Print and shaded views of the part. All mm, measured from the part's lowest x, y and z. Round coordinates to 2 decimals unless told otherwise and drop trailing zeros. Order: outer loops, then holes, each group sorted by start corner. A loop starts at its lowest first (then second) coordinate and runs counter-clockwise, first axis right, second up. Notation, with made-up numbers: (-34, -15) - (-2, -15) arc R27 cw to (-2, 4) - close; hole circle Ø7 at (-0.5, -18). An arc over 180 degrees is marked (long way). Write item = value, one per line. Start each with the question number.
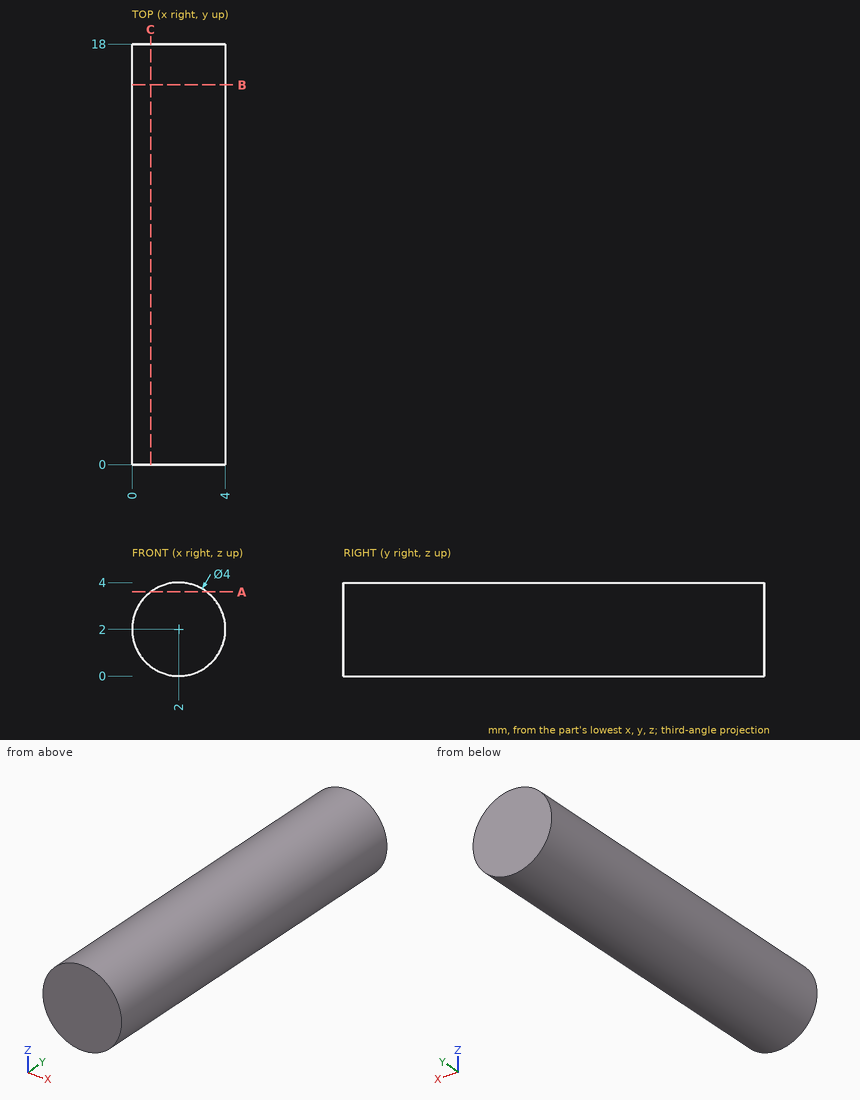
Item 1: Drop a flat-ended pin along its axis: pin 1 (2 mm diameter, centred on x = 0.5, y = 2, fed in from -Z). Give the stop position or say it passes through.
Item 2: Saw through at C-C, the plane x = 0.8. Give the cut face in (y, z), then the cut area to 3 significant figures.
Item 3: Saw through at B-B, the plane y = 16.25. Give the cut face in (x, z).
Item 4: Saw through at A-A, the plane z = 3.6. Give the cut face in (x, y).
Item 5: Probe L1, parallel to X at y = 16.25, z = 2.1; L2, parallel to Z at x = 0.65, y = 7.25; L3, parallel to Z at x = 2.5, y = 16. List the from-to ranges inside material, lowest first.
Check sheet entries:
q1.pin_1 = 0.06
q2.outline = (0, 0.4) - (18, 0.4) - (18, 3.6) - (0, 3.6) - close
q2.area = 57.6 mm2
q3.outline = circle Ø4 at (2, 2)
q4.outline = (0.8, 0) - (3.2, 0) - (3.2, 18) - (0.8, 18) - close
q5.L1 = 0 to 4
q5.L2 = 0.52 to 3.48
q5.L3 = 0.06 to 3.94
